Design review of the part shown in the three views and the two pictorial views. Dimensions are in mm from the part's minimum x, y and z. A direction names the side the tool comes from. Give positions to 0.01 mm unless a question says otherwise; leave off trailing zeros. Order: outer loops, then holes, each group sorted by start corner. A loop starts at its lowest first (then second) coordinate and runs counter-clockwise, first axis right, second up. Notation, with made-up numbers: M 40,0.5 L 79,0.5 A19 ccw 79,19.5 Z; hole C 14,-19.5 d9. An arc over 180 degrees is marked long. Answer as a JSON object with one key per item and string values.
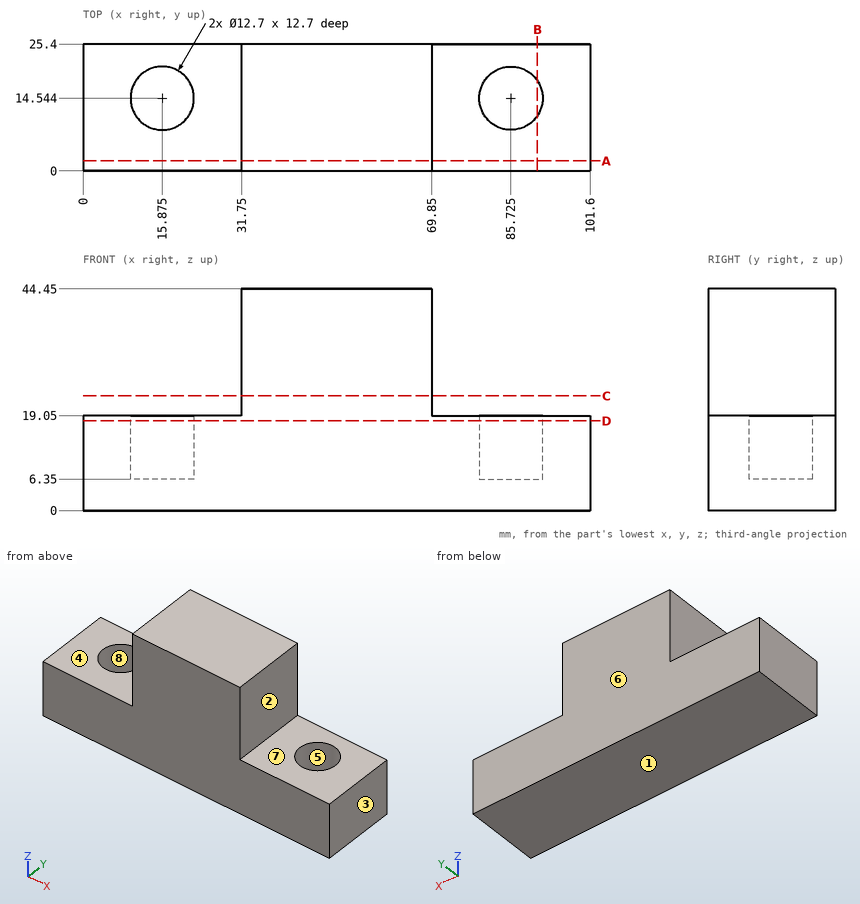
(1) To check wall thickness, follow L1, parallel to X at y = 12.75, z = 8.5; L2, parallel to X at y = 7.5, z = 20; L3, parallel to Z at x = 87.5, y = 3.5. State the ranges of each line that lie inside material, in increasing order. Write a range as from..to.
Checked values:
{"L1": "x = 0..9.78, 21.97..79.63, 91.82..101.6", "L2": "x = 31.75..69.85", "L3": "z = 0..19.05"}
(2) We need section D-D (z = 18). Write out the cut boundary in (x, y) (3 decimals), plus the area to 3 significant figures.
Checked values:
{"outline": "M 0,0 L 101.6,0 L 101.6,25.4 L 0,25.4 Z; hole C 15.875,14.544 d12.7; hole C 85.725,14.544 d12.7", "area": "2,330 mm^2"}
(3) We need section C-C (z = 23). Write out the cut boundary in (x, y), plus the area to 3 significant figures.
Checked values:
{"outline": "M 31.75,0 L 69.85,0 L 69.85,25.4 L 31.75,25.4 Z", "area": "968 mm^2"}
(4) Tool access review of the marked faces 1, 2, 3, 4 and 5: name each direction out of +Z, -Z, +X, -X, +Y, -Y from which nothing blocks a thin tool from reaching the whole face with its end or side.
Checked values:
{"face 1": "-Z, +X, -X, +Y, -Y", "face 2": "+Z, +X, +Y, -Y", "face 3": "+Z, -Z, +X, +Y, -Y", "face 4": "+Z, -X, +Y, -Y", "face 5": "+Z"}
(5) Insertion check: pin 1 (7.5 mm diameter, centred on x = 15.88, y = 14.54, fed in from +Z); pin 2 (2 mm diameter, centred on y = 21, z = 33.5, fed in from -X). Each pin has a flat end and moves straight along its axis. Give the tip position at first contact, or say it passes through.
Checked values:
{"pin 1": "stops at z = 6.35", "pin 2": "stops at x = 31.75"}
(6) We need section B-B (x = 91). Write out the cut boundary in (y, z), plus the area to 3 significant figures.
Checked values:
{"outline": "M 0,0 L 25.4,0 L 25.4,19.05 L 18.08,19.05 L 18.08,6.35 L 11.01,6.35 L 11.01,19.05 L 0,19.05 Z", "area": "394 mm^2"}
(7) We need section A-A (y = 2). Write out the cut boundary in (x, z), plus the area to 3 significant figures.
Checked values:
{"outline": "M 0,0 L 101.6,0 L 101.6,19.05 L 69.85,19.05 L 69.85,44.45 L 31.75,44.45 L 31.75,19.05 L 0,19.05 Z", "area": "2,900 mm^2"}
(8) Draft analysis for pull direction Y (two halves, no side actions). For the marked faces 6, 7 and 8, state which applies: +Y half, -Y half, draft (parallel to the pull), parting line (faces both ways), or undercut.
Checked values:
{"face 6": "+Y half", "face 7": "draft", "face 8": "undercut"}
